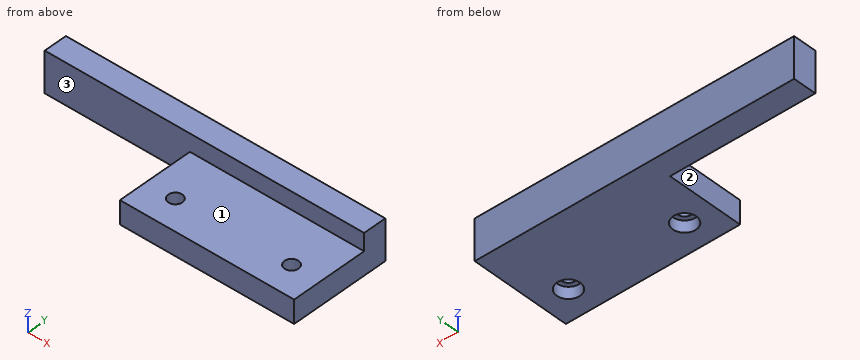
```python
from build123d import *

# Parameters (mm, degrees)
SKETCH_1_W                   = 60
SKETCH_1_H                   = 26.5
EXTRUDE_1_DEPTH              = 8
EXTRUDE_2_DEPTH              = 6
EXTRUDE_2_DEPTH_BACK         = 8
SKETCH_2_W                   = 60
SKETCH_2_H                   = 8
HOLE_WIZARD_M4_1_D           = 4.8
HOLE_WIZARD_M4_1_DEPTH       = 10.1
HOLE_WIZARD_M4_1_CBORE_D     = 8
HOLE_WIZARD_M4_1_CBORE_DEPTH = 4
HOLE_WIZARD_M4_1_TIP         = 1.442065486
SKETCH_7_W                   = 14
SKETCH_7_H                   = 8
EXTRUDE_3_DEPTH              = 50


with BuildPart() as part:
    # 스케치1 → 보스-돌출1 (new body)
    with BuildSketch(Plane.XY):
        Rectangle(SKETCH_1_W, SKETCH_1_H)
    extrude(amount=EXTRUDE_1_DEPTH)

    # 스케치2 → 보스-돌출2 (add, two sides: drawn at the far end of the back side and taken through both)
    with BuildSketch(Plane.XY.offset(8).offset(-EXTRUDE_2_DEPTH_BACK)):
        with Locations((0, 17.25)):
            Rectangle(SKETCH_2_W, SKETCH_2_H)
    extrude(amount=EXTRUDE_2_DEPTH + EXTRUDE_2_DEPTH_BACK)

    # M4 소켓 머리 캡 나사용 카운터보어1
    with Locations(Plane(origin=(0, 0, 0), x_dir=(-1, 0, 0), z_dir=(0, 0, -1))):
        with Locations((-20, -3.25), (20, -3.25)):
            CounterBoreHole(HOLE_WIZARD_M4_1_D / 2, HOLE_WIZARD_M4_1_CBORE_D / 2, HOLE_WIZARD_M4_1_CBORE_DEPTH, depth=HOLE_WIZARD_M4_1_DEPTH)
            with Locations((0, 0, -(HOLE_WIZARD_M4_1_DEPTH + HOLE_WIZARD_M4_1_TIP / 2))):  # 118° drill point
                Cone(0, HOLE_WIZARD_M4_1_D / 2, HOLE_WIZARD_M4_1_TIP, mode=Mode.SUBTRACT)

    # 스케치7 → 보스-돌출3 (add)
    with BuildSketch(Plane.ZY.offset(30)):
        with Locations((7, 17.25)):
            Rectangle(SKETCH_7_W, SKETCH_7_H)
    extrude(amount=EXTRUDE_3_DEPTH)


solid = part.part
```
Geometry: final body of the model. Coordinates: model frame, mm. Face numbers are marked on the shaded views. A direction names the side the tool comes from. Give positions to 0.01 mm unless a question says otherwise; leave off trailing zeros. Write each loop counter-clockwise with the first axis right and the second up, starting at its lowest first coordinate (ties: lowest second). Pieces come first, ordered by that corner, then holes.
1. Pin query (flat end, axial travel): P1, Ø4, axis at y = 5.5, z = 3, coming from the -X side; P2, Ø5, axis at x = -50, z = 3, coming from the -Y side; P3, Ø1.5, axis at x = -8.5, y = 12, coming from the +Z side. Return the tip coordinate at first contact, or that it passes through.
2. Section query C-C, the plane z = 1. Return loops of the section in (x, y).
3. Line query: probe 1 along Y at (x, z) = (20, 6.6); probe 2 along Y at (x, z) = (-20, 1.3); probe 3 along Z at (x, y) = (-2, 3.5). Output: solid intervals per line, ascending.
4. Section query B-B, the plane y = -3.25. Return loops of the section in (x, z).
5. Reachability of the marked faces 1, 2 and 3 from +Z, -Z, +X, -X, +Y, -Y: full face, straight path, thin tool, end or side. Return the list, or none.
6. Section query D-D, the plane x = 8.5. Return loops of the section in (y, z).
7. Section query A-A, the plane x = -20. Return loops of the section in (y, z), then the cut area to 3 significant figures.
Computed:
1. P1: stops at x = -30
1. P2: stops at y = 13.25
1. P3: stops at z = 8
2. outline: (-80, 13.25) - (-30, 13.25) - (-30, -13.25) - (30, -13.25) - (30, 21.25) - (-80, 21.25) - close; hole circle Ø8 at (-20, -3.25); hole circle Ø8 at (20, -3.25)
3. probe 1: y = -13.25 to -5.65, -0.85 to 21.25
3. probe 2: y = -13.25 to -7.25, 0.75 to 21.25
3. probe 3: z = 0 to 8
4. outline: (-30, 0) - (-24, 0) - (-24, 4) - (-22.4, 4) - (-22.4, 8) - (-30, 8) - close; (-17.6, 4) - (-16, 4) - (-16, 0) - (16, 0) - (16, 4) - (17.6, 4) - (17.6, 8) - (-17.6, 8) - close; (22.4, 4) - (24, 4) - (24, 0) - (30, 0) - (30, 8) - (22.4, 8) - close
5. face 1: +Z, +X, -X, -Y
5. face 2: +Z, -Z, -X, -Y
5. face 3: +Z, -X, -Y
6. outline: (-13.25, 0) - (21.25, 0) - (21.25, 14) - (13.25, 14) - (13.25, 8) - (-13.25, 8) - close
7. outline: (-13.25, 0) - (-7.25, 0) - (-7.25, 4) - (-5.65, 4) - (-5.65, 8) - (-13.25, 8) - close; (-0.85, 4) - (0.75, 4) - (0.75, 0) - (21.25, 0) - (21.25, 14) - (13.25, 14) - (13.25, 8) - (-0.85, 8) - close
7. area: 273 mm2
